Read the model definition and answer for the solid it produces. Units are mm, in the model's axes. Coordinates: 2 decimals unless noted, no trailing zeros. Write each loop counter-clockwise with the first axis right and the second up, starting at its lowest first coordinate (ties: lowest second). Pieces come first, ordered by that corner, then holes. Notation, with made-up numbers: (41, 5.5) - (88, 5.5) arc R12 ccw to (88, 23.5) - close; hole circle Ø1 at (78, -4). An arc over 180 degrees is marked (long way). Use a Markdown table: item, result.
from build123d import *

# Parameters (mm, degrees)
F0_W     = 80
F0_H     = 80
F0_R     = 2
F1_DEPTH = 25.5
F2_R     = 5
F3_R     = 39
F4_DEPTH = 25.5


with BuildPart() as f1:
    # F0 (on Front) → F1 (new body)
    with BuildSketch(Plane.XZ):
        with Locations((78.061389, -1.505866)):
            Rectangle(F0_W, F0_H)
        with Locations((42.311389, -37.255866)):
            Circle(F0_R, mode=Mode.SUBTRACT)
        with Locations((113.811389, -37.255866)):
            Circle(F0_R, mode=Mode.SUBTRACT)
        with Locations((42.311389, 34.244134)):
            Circle(F0_R, mode=Mode.SUBTRACT)
        with Locations((113.811389, 34.244134)):
            Circle(F0_R, mode=Mode.SUBTRACT)
    extrude(amount=F1_DEPTH)

    # F2
    f2_edges = [f1.edges().sort_by_distance(p)[0] for p in [
        (38.061389, -12.75, 38.494134),
        (38.061389, -12.75, -41.505866),
        (118.061389, -12.75, -41.505866),
        (118.061389, -12.75, 38.494134),
    ]]
    fillet(f2_edges, radius=F2_R)

    # F3 (on face) → F4 (cut, through all)
    with BuildSketch(Plane.XZ.offset(25.5)):
        with Locations((78.061389, -1.505866)):
            Circle(F3_R)
    extrude(amount=-F4_DEPTH, mode=Mode.SUBTRACT)


solid = f1.part
(1) The mould has two halves that part along X. Classify faces 1 (the cylindrical face through (39.487, -12.928, 36.991)), 2 (the cylindrical face through (41.88, -12.57, -39.21)), 3 (the cylindrical face through (116.558, -12.928, 37.068)): pulls with the +X half, pulls with the -X half, needs draft (parallel to the pull), parting line crosses it, or undercut.
Report:
| item | result |
|---|---|
| face 1 | pulls with the -X half |
| face 2 | undercut |
| face 3 | pulls with the +X half |
(2) A cutting plane is placed at A-A, the plane x = 88.5. Write down the section's boundary in (y, z), and give its area (3 significant figures).
Report:
| item | result |
|---|---|
| outline | (-25.5, -41.51) - (0, -41.51) - (0, -39.08) - (-25.5, -39.08) - close; (-25.5, 36.07) - (0, 36.07) - (0, 38.49) - (-25.5, 38.49) - close |
| area | 124 mm² |
(3) A cutting plane is placed at C-C, the plane y = -4.5. Write down the section's boundary in (x, z).
Report:
| item | result |
|---|---|
| outline | (38.06, -36.51) arc R5 ccw to (43.06, -41.51) - (113.06, -41.51) arc R5 ccw to (118.06, -36.51) - (118.06, 33.49) arc R5 ccw to (113.06, 38.49) - (43.06, 38.49) arc R5 ccw to (38.06, 33.49) - close; hole circle Ø78 at (78.06, -1.51); hole circle Ø4 at (42.31, -37.26); hole circle Ø4 at (42.31, 34.24); hole circle Ø4 at (113.81, -37.26); hole circle Ø4 at (113.81, 34.24) |
(4) A cutting plane is placed at B-B, the plane z = 12. Write down the section's boundary in (x, y).
Report:
| item | result |
|---|---|
| outline | (38.06, -25.5) - (41.47, -25.5) - (41.47, 0) - (38.06, 0) - close; (114.65, -25.5) - (118.06, -25.5) - (118.06, 0) - (114.65, 0) - close |
(5) Straight lines are drawn through the part: L1, parallel to X at y = -5.75, z = -1; L2, parallel to Z at x = 77, y = -16.75; L3, parallel to Z at x = 91, y = -9.75. For each, find the intervals that lie inside material, in ascending order.
Report:
| item | result |
|---|---|
| L1 | x = 38.06 to 39.06, 117.06 to 118.06 |
| L2 | z = -41.51 to -40.49, 37.48 to 38.49 |
| L3 | z = -41.51 to -38.3, 35.29 to 38.49 |
